from build123d import *

# Parameters (mm, degrees)
SKETCH_1_W      = 74.6
SKETCH_1_H      = 95.1
SKETCH_1_R      = 1.5
EXTRUDE_1_DEPTH = 3
EXTRUDE_2_DEPTH = 1
SKETCH_3_R      = 5
EXTRUDE_3_DEPTH = 1
SKETCH_4_W      = 2.4
SKETCH_4_H      = 76
SKETCH_4_W_2    = 5.142957709
SKETCH_4_H_2    = 9.820324755
EXTRUDE_4_DEPTH = 2


with BuildPart() as part:
    # 草图1 → 凸台-拉伸1 (new body)
    with BuildSketch(Plane(origin=(0, 0, 0), x_dir=(1, 0, 0), z_dir=(0, 1, 0))):
        Rectangle(SKETCH_1_W, SKETCH_1_H)
        with Locations(Location((-34.225, -40.515, 0), (0, 0, 270))):
            Circle(SKETCH_1_R, mode=Mode.SUBTRACT)
        with Locations(Location((-34.225, 44.515, 0), (0, 0, 270))):
            Circle(SKETCH_1_R, mode=Mode.SUBTRACT)
        with Locations(Location((34.225, 44.515, 0), (0, 0, 270))):
            Circle(SKETCH_1_R, mode=Mode.SUBTRACT)
        with Locations(Location((34.225, -40.515, 0), (0, 0, 270))):
            Circle(SKETCH_1_R, mode=Mode.SUBTRACT)
    extrude(amount=EXTRUDE_1_DEPTH)

    # 草图2 → 凸台-拉伸2 (add)
    with BuildSketch(Plane(origin=(0, 3, 0), x_dir=(1, 0, 0), z_dir=(0, 1, 0))):
        Polygon((-9.889416187, 3.833985847), (-3.833985847, -9.889416187), (9.889416187, -3.833985847), (3.833985847, 9.889416187), align=None)
    extrude(amount=EXTRUDE_2_DEPTH)

    # 草图3 → 凸台-拉伸3 (add)
    with BuildSketch(Plane(origin=(0, 3, 0), x_dir=(1, 0, 0), z_dir=(0, 1, 0))):
        with Locations(Location((-23.440659091, -26.14028556, 0), (0, 0, 270))):
            Circle(SKETCH_3_R)
    extrude(amount=EXTRUDE_3_DEPTH)

    # 草图4 → 凸台-拉伸4 (add)
    with BuildSketch(Plane(origin=(0, 3, 0), x_dir=(1, 0, 0), z_dir=(0, 1, 0))):
        with Locations((-32.5, 3.325457596)):
            Rectangle(SKETCH_4_W, SKETCH_4_H)
        with Locations((27.55007403, 41.325457596)):
            Rectangle(SKETCH_4_W_2, SKETCH_4_H_2)
    extrude(amount=EXTRUDE_4_DEPTH)


solid = part.part
Check sheet for the modelled part. Datum: model origin and axes. Units: mm. A direction names the side the tool comes from. Give positions to 0.01 mm unless a question says otherwise; leave off trailing zeros. Order: outer loops, then holes, each group sorted by start corner. A loop starts at its lowest first (then second) coordinate and runs counter-clockwise, first axis right, second up. Notation, with made-up numbers: M -30.75,-6 L -18.75,-6 A14 cw -18.75,1 Z; hole C 12.5,13.5 d2. An arc over 180 degrees is marked long. Answer as CSV lines item,"result". Start each with the question number.
Item 1: Cross-section at A-A on z = -17.5. Enter the section's corners in (x, y), plus the area to 3 significant figures.
Item 2: Cross-section at B-B on x = -24.5. Enter the section's corners in (y, z), plus the area to 3 significant figures.
Item 3: Mould release check, pull along Z, two halves, no side actions. Record for faces 4 (the face through (34.676, 1.479, -43.084)), 5 (the face through (37.3, 1, 1)), 6 (the face through (-33, 4, 34.675)), 7 (the face through (-34.8, 1.48, -43.13)): +Z half, -Z half, draft (parallel to the pull), parting line (faces both ways), or undercut.
Item 4: Thickness scan on line 1 (Y direction, x = 12, z = 28); line 2 (X direction, y = 3.9, z = -3); line 3 (Y direction, x = 2.5, z = -8). Record the ranges inside material, lowest first. Write a range as [from, to].
Item 5: Tool access check on faces 1 (the face through (-31.3, 4, -3)), 2 (the face through (-33.7, 4, -3)), 3 (the face through (2.932, 3.493, 6.904)). Record the directions out of +Z, -Z, +X, -X, +Y, -Y that give a thin tool (end or side, any length) a straight path to the whole face; none if there is none.
Item 6: Gauge pin test, flat ends, axial feed: P1, Ø11, axis at x = -22.5, z = 25, coming from the +Y side; P2, Ø1.6, axis at x = 28.5, y = 4.5, coming from the -Z side; P3, Ø0.6, axis at x = -33, y = 3.5, coming from the +Z side; P4, Ø2.5, axis at x = 34.225, z = -44.515, coming from the +Y side. Record the tip position at first contact, or that the pin passes through.
Item 7: Cross-section at D-D on x = -12.5. Enter the section's corners in (y, z).
Item 8: Cross-section at C-C on z = -39. Enter the section's corners in (x, y).
Established:
1,outline,"M -37.3,0 L 37.3,0 L 37.3,3 L -31.3,3 L -31.3,5 L -33.7,5 L -33.7,3 L -37.3,3 Z"
1,area,"229 mm^2"
2,outline,"M 0,-47.55 L 3,-47.55 L 3,21.25 L 4,21.25 L 4,31.03 L 3,31.03 L 3,47.55 L 0,47.55 Z"
2,area,"295 mm^2"
3,face 4,"undercut"
3,face 5,"draft"
3,face 6,"+Z half"
3,face 7,"undercut"
4,line 1,"y = [0, 3]"
4,line 2,"x = [-33.7, -31.3], [-9.52, 6.87]"
4,line 3,"y = [0, 4]"
5,face 1,"+Z, -Z, +Y"
5,face 2,"+Z, -Z, -X, +Y"
5,face 3,"+Z, +X, +Y"
6,P1,"stops at y = 4"
6,P2,"stops at z = -46.24"
6,P3,"stops at z = 34.67"
6,P4,"passes through"
7,outline,"M 0,-47.55 L 3,-47.55 L 3,47.55 L 0,47.55 Z"
8,outline,"M -37.3,0 L 37.3,0 L 37.3,3 L 30.12,3 L 30.12,5 L 24.98,5 L 24.98,3 L -31.3,3 L -31.3,5 L -33.7,5 L -33.7,3 L -37.3,3 Z"
